Print and shaded views of the part. All mm, measured from the part's lowest x, y and z. Give positions to 0.01 mm unless a question says otherwise; leave off trailing zeros. Loops run counter-clockwise (first coordinate to the right, second up) from the corner with the lowest first, then second, coordinate; pieces in that order, holes last. Notation, with made-up numbers: (21, 66) - (50, 66) arc R7 cw to (50, 74) - close; hole circle Ø6 at (-5, 81). An arc over 180 degrees is marked (long way). Return JSON: item names as keys, results as strings.
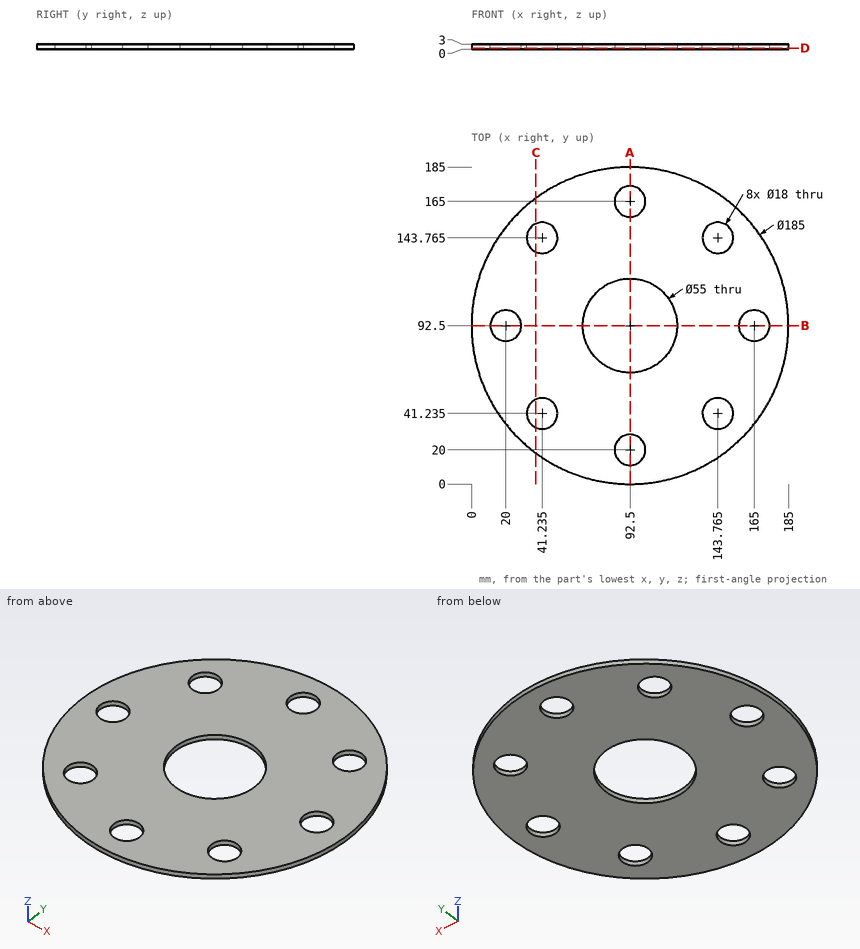
1. Cut at C-C, the plane x = 37.5. Write the cut outline in (y, z).
Values follow:
{"outline": "(18.13, 0) - (33.05, 0) - (33.05, 3) - (18.13, 3) - close; (49.42, 0) - (135.58, 0) - (135.58, 3) - (49.42, 3) - close; (151.95, 0) - (166.87, 0) - (166.87, 3) - (151.95, 3) - close"}
2. Drop a flat-ended pin along its axis: P1, Ø1.5, axis at x = 130, z = 1.5, coming from the +Y side. Give the stop position or say it passes through.
Values follow:
{"P1": "stops at y = 177.39"}
3. Drill centre lines: probe 1 along Y at (x, z) = (92.5, 2.45); probe 2 along X at (y, z) = (142.5, 0.55) (1 decimal); probe 3 along X at (y, z) = (135.5, 2) (1 decimal). Where is each one in solid material? Low to high.
Values follow:
{"probe 1": "y = 0 to 11, 29 to 65, 120 to 156, 174 to 185", "probe 2": "x = 14.7 to 32.3, 50.1 to 134.9, 152.7 to 170.3", "probe 3": "x = 10.6 to 37.7, 44.8 to 140.2, 147.3 to 174.4"}
4. Cut at A-A, the plane x = 92.5. Write the cut outline in (y, z).
Values follow:
{"outline": "(0, 0) - (11, 0) - (11, 3) - (0, 3) - close; (29, 0) - (65, 0) - (65, 3) - (29, 3) - close; (120, 0) - (156, 0) - (156, 3) - (120, 3) - close; (174, 0) - (185, 0) - (185, 3) - (174, 3) - close"}
5. Cut at D-D, the plane z = 0.55. Give the number of separate pieces and of enclosed holes in the cut face, plus the area to 3 significant figures.
Values follow:
{"separate pieces": "1", "enclosed holes": "9", "area": "22,500 mm²"}
